Design review of the part built by this model. Coordinates are the model's own, in mm. A direction names the side the tool comes from. Coordinates: 2 decimals unless noted, no trailing zeros. Loops run counter-clockwise (first coordinate to the right, second up) from the corner with the lowest first, then second, coordinate; pieces in that order, holes last. Notation, with made-up numbers: (39.5, 48.5) - (50.5, 48.5) arc R20 cw to (50.5, 54.5) - close; hole circle Ø11 at (35, 68.25). An arc over 180 degrees is marked (long way). Use one line per item in the form item = value. Start each with the question number.
(1) The part is to be moulded in two halves that separate along X. For faces 4 (the face through (13, -5, 6)), 5 (the face through (5, -7, 8)), 6 (the face through (12.548, 4.972, 8.581)), say which applies: pulls with the +X half, pulls with the -X half, needs draft (parallel to the pull), parting line crosses it, or undercut.
(2) Add section B-B (x = -1.5). State the section outline as (y, z) points, plus the area to 3 significant figures.
(3) Tool access review of faces 1 (the face through (2, -5, 9)), 2 (the face through (8.693, -5.028, 8.8)), 3 (the face through (2, 4, 9)): name each direction out of +Z, -Z, +X, -X, +Y, -Y from which nothing blocks a thin tool from reaching the whole face with its end or side.
(4) For L1, parallel to Y at x = -1.5, z = 1.15; L2, parallel to Y at x = 14, z = 10.5; L3, parallel to Z at x = -1, y = 6, list the stretches that pass through material, from the lowest coordinate up.
(5) Clearance check with flat-ended pins moving along their axes: pin 1 Ø3 at (x, z) = (-1, 10.5) entering from +Y; pin 2 Ø2 at (x, y) = (7, 4) entering from -Z; pin 3 Ø5.5 at (x, y) = (-2, 5.5) entering from +Z. State where each tip first meets the part, or that it passes through.
(6) Add section D-D (x = 5.75). State the section outline as (y, z) points.
(7) Add section C-C (z = 1.5). State the section outline as (x, y) points, plus the area to 3 significant figures.
(8) Add section A-A (y = 4). State the section outline as (x, z) points, plus the area to 3 significant figures.
```python
from build123d import *

# Parameters (mm, degrees)
SKETCH_1_W          = 10
SKETCH_1_H          = 14
EXTRUDE_1_DEPTH     = 3
SKETCH_2_W          = 3
SKETCH_2_H          = 14
EXTRUDE_2_DEPTH     = 12
RIB_1_REACH         = 19.292
SKETCH_3_WALL_W     = 50.475676922
SKETCH_3_WALL_H     = 3
HOLE_WIZARD_M3_2_D  = 2.5
SKETCH_7_W          = 10
SKETCH_7_H          = 4
EXTRUDE_3_DEPTH     = 10
FILLET_1_R          = 1
FILLET_2_R          = 0.5
FILLET_3_R          = 1
SKETCH_8_R          = 2.6
CUT_EXTRUDE_3_DEPTH = 4
HOLE_WIZARD_M5_1_D  = 4.2
FILLET_5_R          = 5


with BuildPart() as part:
    # 草图1 → 凸台-拉伸1 (new body)
    with BuildSketch(Plane.XY):
        Rectangle(SKETCH_1_W, SKETCH_1_H)
    extrude(amount=EXTRUDE_1_DEPTH)

    # 草图2 → 凸台-拉伸2 (add)
    with BuildSketch(Plane.XY.offset(3)):
        with Locations((3.5, 0)):
            Rectangle(SKETCH_2_W, SKETCH_2_H)
    extrude(amount=EXTRUDE_2_DEPTH)

    # 草图3 wall → 筋1 (add, up to next)
    with BuildSketch(Plane(origin=(-1.5, 0, 9), x_dir=(0.503871025524, 0, 0.863778900898), z_dir=(-0.863778900898, 0, 0.503871025524)), mode=Mode.PRIVATE) as rib_1_sk1:
        Rectangle(SKETCH_3_WALL_W, SKETCH_3_WALL_H)
    rib_1_tool1 = extrude(rib_1_sk1.sketch, amount=-RIB_1_REACH, mode=Mode.PRIVATE) - part.part
    add(rib_1_tool1.solids().sort_by_distance((-1.5, 0, 9))[0])

    # M3 螺纹孔2 (through all)
    with Locations(Plane(origin=(-1.5, 4, 3), x_dir=(1, 0, 0), z_dir=(0, 0, 1))):
        with Locations((0, 0), (0, -8)):
            Hole(HOLE_WIZARD_M3_2_D / 2)

    # 草图7 → 凸台-拉伸3 (add)
    with BuildSketch(Plane(origin=(5, 0, 0), x_dir=(0, 0, -1), z_dir=(1, 0, 0))):
        with Locations((-10, -5)):
            Rectangle(SKETCH_7_W, SKETCH_7_H)
        with Locations((-10, 5)):
            Rectangle(SKETCH_7_W, SKETCH_7_H)
    extrude(amount=EXTRUDE_3_DEPTH)

    # 圆角1
    fillet_1_edges = [part.edges().sort_by_distance(p)[0] for p in [
        (15, -5, 15),
        (15, 5, 15),
    ]]
    fillet(fillet_1_edges, radius=FILLET_1_R)

    # 圆角2
    fillet_2_edges = [part.edges().sort_by_distance(p)[0] for p in [
        (2, -1.5, 9),
        (-1.5, 1.5, 3),
        (-1.5, -1.5, 3),
        (2, 1.5, 9),
    ]]
    fillet(fillet_2_edges, radius=FILLET_2_R)

    # 圆角3
    fillet_3_edges = [part.edges().sort_by_distance(p)[0] for p in [
        (-5, -7, 1.5),
        (-5, 7, 1.5),
    ]]
    fillet(fillet_3_edges, radius=FILLET_3_R)

    # 草图8 → 切除-拉伸3 (cut)
    with BuildSketch(Plane.XZ.offset(7)):
        with Locations(Location((11, 10, 0), (0, 0, 270))):
            Circle(SKETCH_8_R)
    extrude(amount=-CUT_EXTRUDE_3_DEPTH, mode=Mode.SUBTRACT)

    # M5 螺纹孔1 (through all)
    with Locations(Plane(origin=(0, 7, 0), x_dir=(1, 0, 0), z_dir=(0, 1, 0))):
        with Locations((11, -10)):
            Hole(HOLE_WIZARD_M5_1_D / 2)

    # 圆角5
    fillet_5_edges = [part.edges().sort_by_distance(p)[0] for p in [
        (15, -5, 5),
        (15, 5, 5),
    ]]
    fillet(fillet_5_edges, radius=FILLET_5_R)


solid = part.part
```
Computed values:
q1.face_4 = pulls with the +X half
q1.face_5 = needs draft
q1.face_6 = undercut
q2.outline = (-7, 0) - (-5.25, 0) - (-5.25, 3) - (-7, 3) - close; (-2.75, 0) - (2.75, 0) - (2.75, 3) - (2, 3) arc R0.5 cw to (1.5, 3.5) - (1.5, 9) - (-1.5, 9) - (-1.5, 3.5) arc R0.5 cw to (-2, 3) - (-2.75, 3) - close; (5.25, 0) - (7, 0) - (7, 3) - (5.25, 3) - close
q2.area = 45.1 mm^2
q3.face_1 = +Z, -X, -Y
q3.face_2 = -Y
q3.face_3 = +Z, -X, +Y
q4.L1 = -7 to -5.25, -2.75 to 2.75, 5.25 to 7
q4.L2 = -7 to -3, 3 to 7
q4.L3 = 0 to 3
q5.pin_1 = 1.5
q5.pin_2 = 5
q5.pin_3 = 3
q6.outline = (-7, 5) - (-3, 5) - (-3, 15) - (-7, 15) - close; (3, 5) - (7, 5) - (7, 15) - (3, 15) - close
q7.outline = (-5, -6) arc R1 ccw to (-4, -7) - (5, -7) - (5, 7) - (-4, 7) arc R1 ccw to (-5, 6) - close; hole circle Ø2.5 at (-1.5, -4); hole circle Ø2.5 at (-1.5, 4)
q7.area = 130 mm^2
q8.outline = (-5, 0) - (-2.75, 0) - (-2.75, 3) - (-5, 3) - close; (-0.25, 0) - (5, 0) - (5, 5) - (10, 5) arc R5 ccw to (15, 10) - (15, 14) arc R1 ccw to (14, 15) - (2, 15) - (2, 3) - (-0.25, 3) - close; hole circle Ø4.2 at (11, 10)
q8.area = 139 mm^2
